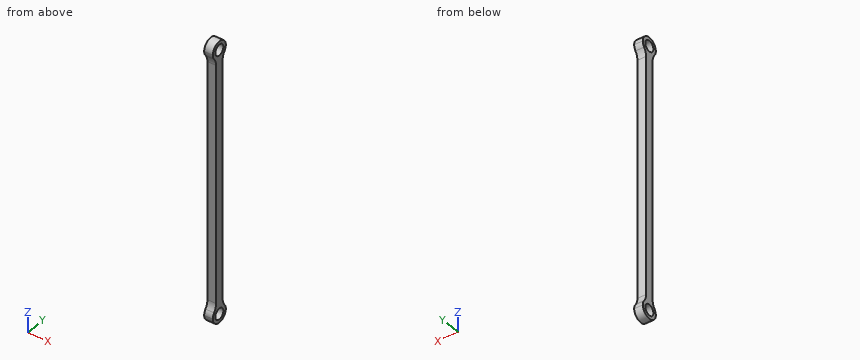
from build123d import *
from build123d.topology import SkipClean

# Parameters (mm, degrees)
SKETCH_1_R          = 5
EXTRUDE_1_DEPTH     = 8
CUT_EXTRUDE_1_DEPTH = 253.753338257
FILLET_1_R          = 12


with BuildPart() as part:
    # 草图1 → 凸台-拉伸1 (new body)
    with BuildSketch(Plane(origin=(0, 0, 0), x_dir=(0, 0, -1), z_dir=(1, 0, 0))):
        with BuildLine():
            Line((0, 8), (244.5, 8))
            ThreePointArc((244.5, 8), (252.5, 0), (244.5, -8))
            Line((244.5, -8), (0, -8))
            ThreePointArc((0, -8), (-8, 0), (0, 8))
        make_face()
        with Locations((244.5, 0)):
            Circle(SKETCH_1_R, mode=Mode.SUBTRACT)
        Circle(SKETCH_1_R, mode=Mode.SUBTRACT)
    extrude(amount=EXTRUDE_1_DEPTH)

    # 草图2 → 切除-拉伸1 (cut, through all)
    with SkipClean():  # the faces are left unmerged after this step: merging them gives an invalid solid
        with BuildSketch(Plane(origin=(8, 0, 0), x_dir=(0, 0, -1), z_dir=(1, 0, 0))):
            with BuildLine():
                Line((237.57179677, -4), (6.92820323, -4))
                ThreePointArc((6.92820323, -4), (4, -6.92820323), (0, -8))
                Line((0, -8), (244.5, -8))
                ThreePointArc((244.5, -8), (240.5, -6.92820323), (237.57179677, -4))
            make_face()
            with BuildLine():
                Line((237.57179677, 4), (6.92820323, 4))
                ThreePointArc((6.92820323, 4), (4, 6.92820323), (0, 8))
                Line((0, 8), (244.5, 8))
                ThreePointArc((244.5, 8), (240.5, 6.92820323), (237.57179677, 4))
            make_face()
        extrude(amount=-CUT_EXTRUDE_1_DEPTH, mode=Mode.SUBTRACT)

    # 圆角1
    fillet_1_edges = [part.edges().sort_by_distance(p)[0] for p in [
        (4, -4, -6.92820323),
        (4, -4, -237.57179677),
        (4, 4, -237.57179677),
        (4, 4, -6.92820323),
    ]]
    fillet(fillet_1_edges, radius=FILLET_1_R)


with BuildPart() as part_1:
    # Move Body 5: moved
    add(part.part.moved(Location((0, 0, 244.5))))


with BuildPart() as part_2:
    # Move Body 3: moved
    add(part_1.part.moved(Location((0, 0, -244.5))))


solid = part_2.part
Design review of the part built by this model. Coordinates are the model's own, in mm. Round coordinates to 2 decimals unless told otherwise and drop trailing zeros. Loops run counter-clockwise (first coordinate to the right, second up) from the corner with the lowest first, then second, coordinate; pieces in that order, holes last. Notation, with made-up numbers: (49.25, 28) - (73.25, 28) arc R26 cw to (73.25, 58) - close; hole circle Ø4 at (14, 81). An arc over 180 degrees is marked (long way). One line per item, written item: value. Start each with the question number.
1) Consider section C-C on z = -193. Give the boundary of the cut face in (x, y).
2) Consider section B-B on x = 5. Give the boundary of the cut face in (y, z), then the cut area to 3 significant figures.
3) Consider section A-A on y = 0. Give the boundary of the cut face in (x, z), then the cut area to 3 significant figures.
4) To check wall thickness, follow L1, parallel to Z at x = 5, y = -0.5; L2, parallel to Y at x = 5, z = 0; L3, parallel to Z at x = 7.25, y = 2.5. State the ranges of each line that lie inside material, in increasing order. Write a range as from..to.
5) Insertion check: pin 1 Ø1 at (x, y) = (5.5, -3) entering from +Z; pin 2 Ø4 at (x, z) = (3.5, -117.5) entering from -Y; pin 3 Ø1.5 at (x, z) = (4, -214) entering from +Y. Each pin has a flat end and moves straight along its axis. Give the tip position at first contact, or say it passes through.
Reported:
1. outline: (0, -4) - (8, -4) - (8, 4) - (0, 4) - close
2. outline: (-6.4, -239.7) arc R8 ccw (long way) to (6.4, -239.7) arc R12 cw to (4, -232.5) - (4, -12) arc R12 cw to (6.4, -4.8) arc R8 ccw (long way) to (-6.4, -4.8) arc R12 cw to (-4, -12) - (-4, -232.5) arc R12 cw to start; hole circle Ø10 at (0, -244.5); hole circle Ø10 at (0, 0)
2. area: 2,090 mm^2
3. outline: (0, -252.5) - (8, -252.5) - (8, -249.5) - (0, -249.5) - close; (0, -239.5) - (8, -239.5) - (8, -5) - (0, -5) - close; (0, 5) - (8, 5) - (8, 8) - (0, 8) - close
3. area: 1,920 mm^2
4. L1: z = -252.48..-249.47, -239.53..-4.97, 4.97..7.98
4. L2: y = -8..-5, 5..8
4. L3: z = -252.1..-248.83, -240.17..-4.33, 4.33..7.6
5. pin 1: stops at z = 7.6
5. pin 2: stops at y = -4
5. pin 3: stops at y = 4
